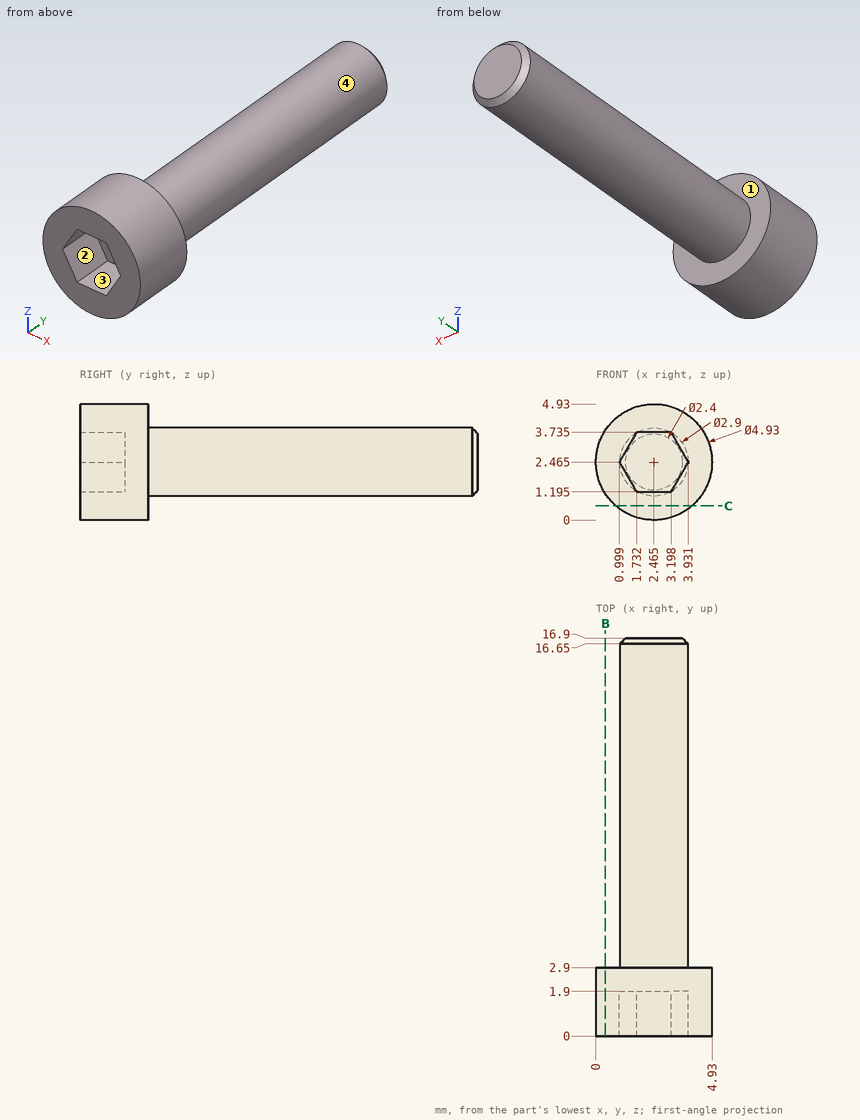
Part print with two shaded views. Sizes in mm from the minimum x, y, z corner. Round coordinates to 2 decimals unless told otherwise and drop trailing zeros. Order: outer loops, then holes, each group sorted by start corner. A loop starts at its lowest first (then second) coordinate and runs counter-clockwise, first axis right, second up. Notation, with made-up numbers: (19.25, -14.5) -> (56.25, -14.5) arc R27 ccw to (56.25, 24.5) -> close; hole circle Ø5 at (43.5, 67). An arc over 180 degrees is marked (long way). Use one line per item in the form item = value.
Item 1: Cut at B-B, the plane x = 0.4. Write the cut outline in (y, z).
Returned:
outline = (0, 1.12) -> (2.9, 1.12) -> (2.9, 3.81) -> (0, 3.81) -> close
Item 2: Drill centre lines: line 1 (Y direction, x = 4.45, z = 2.25); line 2 (X direction, y = 7, z = 2.45) (1 decimal); line 3 (Z direction, x = 2.7, y = 1.5) (1 decimal). Where is each one in solid material? Low to high.
Returned:
line_1 = 0 to 2.9
line_2 = 1 to 3.9
line_3 = 0 to 1.2, 3.7 to 4.9
Item 3: Flat gauge pins, fed straight in: pin 1 Ø0.8 at (x, z) = (2.5, 3) entering from -Y; pin 2 Ø1.5 at (x, y) = (2, 5.5) entering from -Z (3 decimals). Where does each tip first touch, or does it go through?
Returned:
pin_1 = 1.9
pin_2 = 1.015
Item 4: Pull direction X, two halves, no side cores. Call the marked faces 1, 2, 3 and 4: released by +X, released by -X, zero draft, split by the parting line, or undercut.
Returned:
face_1 = zero draft
face_2 = undercut
face_3 = undercut
face_4 = split by the parting line
Item 5: Cut at C-C, the plane z = 0.6. Write the cut outline in (x, y).
Returned:
outline = (0.85, 0) -> (4.08, 0) -> (4.08, 2.9) -> (0.85, 2.9) -> close
